```python
from build123d import *

# Parameters (mm, degrees)
F3_R = 2.1064176113
F4_R = 5


# Not quite as in the source:
# - a fillet or chamfer that OpenCascade refuses, or shapes differently, is made with other operations: its cross-section is extruded or revolved along the edge and cut away or added


with BuildPart() as f1:
    # F0 (on Front) → F1 (revolve)
    with BuildSketch(Plane.XZ):
        Polygon((-10.9814703465, 0), (0, 0), (0, 22.2597364336), (-4.8476760276, 22.2597364336), (-6.4305909909, 19.6906365962), (-9.2006912455, 19.6906365962), (-10.9814703465, 21.8640081584), (-19.5646515468, 21.8640081584), (-19.5646515468, 19.6906365962), (-10.9814703465, 16.7195349932), (-14.5430285484, 6.4305905253), align=None)
    revolve(axis=Axis((0, 0, 11.1298682168), (0, 0, -1)))

    # F2: fillet of radius 10.1048761085 on 1 edges, made by hand

    # F2_s1 → F2_t2 (revolve, cut)
    with BuildSketch(Plane.XZ):
        with BuildLine():
            ThreePointArc((-19.5646515468, 21.8640081584), (-17.3375812271, 19.4776240652), (-14.4659586897, 17.9257042049))
            Line((-14.4659586897, 17.9257042049), (-19.5646515468, 19.6906365962))
            Line((-19.5646515468, 19.6906365962), (-19.5646515468, 21.8640081584))
        make_face()
    revolve(axis=Axis((0, 0, 19.6906365962), (0, 0, -1)), mode=Mode.SUBTRACT)

    # F3
    f3_edges = [f1.edges().sort_by_distance(p)[0] for p in [
        (14.543029, 0, 6.430591),
    ]]
    fillet(f3_edges, radius=F3_R)

    # F4
    f4_edges = [f1.edges().sort_by_distance(p)[0] for p in [
        (10.98147, 0, 21.864008),
        (4.847676, 0, 22.259736),
    ]]
    fillet(f4_edges, radius=F4_R)


solid = f1.part
```
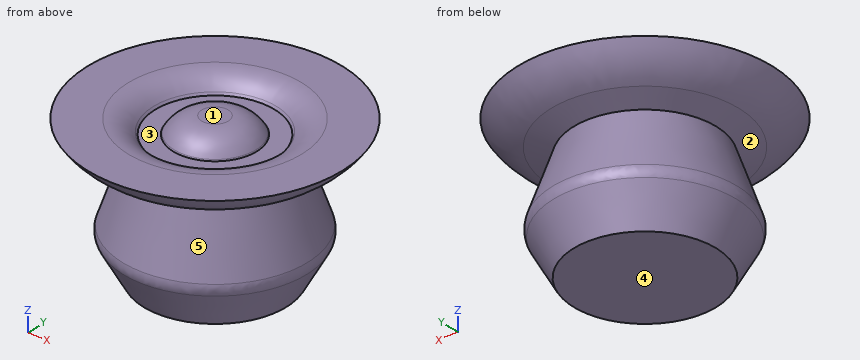
Can you work these out from the model? Positions are in its coordinate system, mm. Face numbers are marked on the shaded views. A direction names the side the tool comes from. Round coordinates to 2 decimals unless told otherwise and drop trailing zeros. Loops run counter-clockwise (first coordinate to the right, second up) from the corner with the lowest first, then second, coordinate; pieces in that order, holes last. Notation, with made-up numbers: M -27,-5 L -13,-5 A26 ccw -13,28 Z; hole C 27,73.25 d7. An arc over 180 degrees is marked long. Write item = value, one per line. Start each with the question number.
(1) I'm going to push flat-ended pins straight in: P1, Ø4, axis at y = -9.5, z = 10, coming from the -X side; P2, Ø1, axis at y = -15.5, z = 3.5, coming from the +X side; P3, Ø12, axis at x = 9, z = 7.5, coming from the -Y side; P4, Ø2, axis at x = 8, z = 3.5, coming from the +Y side. Where does each tip first touch, or does it pass through?
(2) Suppose I cut it at B-B on z = 8.5. Write out the boundary of the cut face in (x, y).
(3) Which directions (+Z, -Z, +X, -X, +Y, -Y) give clear straight access to the entire face, cutting with the end or side of a thin tool? Please do the marked faces 4 and 5.
(4) I need wall thicknesses on line 1 along Z through (x, y) = (-2, 6.5); line 2 along X through (y, z) = (-6, 9); line 3 along Y through (x, z) = (-6.5, 5.75). Which ranges of each line are inside material? Lowest first, please.
(5) Suppose I cut it at A-A on z = 12. Write out the boundary of the cut face in (x, y), plus the area to 3 significant figures.
(6) If we mould it in two halves opening along Y, with no side actions, what happens to the marked faces 1, 2 and 3? For each: released by +Y, released by -Y, zero draft, split by the parting line, or undercut.
Answer block:
q1.P1 = -11.23
q1.P2 = through
q1.P3 = -14.02
q1.P4 = 11.14
q2.outline = C 0,0 d27.65
q3.face_4 = -Z, +X, -X, +Y, -Y
q3.face_5 = none
q4.line_1 = 0 to 19.69
q4.line_2 = -12.26 to 12.26
q4.line_3 = -12.58 to 12.58
q5.outline = C 0,0 d25.23
q5.area = 500 mm²
q6.face_1 = zero draft
q6.face_2 = split by the parting line
q6.face_3 = undercut
